Verification items for this drawing (mm, ordinates from the low corner). A direction names the side the tool comes from. Give positions to 0.01 mm unless a question says otherwise; leave off trailing zeros. Loops run counter-clockwise (first coordinate to the right, second up) from the corner with the lowest first, then second, coordinate; pieces in that order, holes last. Notation, with made-up numbers: (86.5, -5.75) -> (103.5, -5.75) arc R12 ccw to (103.5, 13.25) -> close; hole circle Ø4 at (-6.5, 81.5). An arc over 180 degrees is marked (long way). Write each question's results on one line, items separated by ' | '. Start each with the question number.
Item 1: Access from +Z, -Z, +X, -X, +Y, -Y to the whole of each face (thin tool, end or side, straight path). Record for the marked faces 1 and 2.
Item 2: Gauge pin test, flat end, axial feed: pin 1 Ø3 at (x, z) = (11, 19.5) entering from -Y. Record the tip position at first contact, or that the pin passes through.
Item 3: Mould release check, pull along Z, two halves, no side actions. Record for the marked faces 3, 4, 5 and 6: pulls with the +Z half, pulls with the -Z half, needs draft (parallel to the pull), parting line crosses it, or undercut.
Item 4: Cross-section at A-A on x = 12.5. Enter the section's corners in (y, z).
Item 5: Scan lines: line 1 along X through (y, z) = (6.35, 17.5); line 2 along X through (y, z) = (1.45, 17.5); line 3 along Z through (x, y) = (27.5, 2.5). Record each from-to range of solid material in increasing order.
Item 6: Cross-section at C-C on y = 0.5. Enter the section's corners in (x, z).
Item 7: Cross-section at B-B on z = 16.5. Enter the section's corners in (x, y).
Item 8: Cross-section at D-D on y = 7.75. Enter the section's corners in (x, z), then the cut area to 3 significant figures.
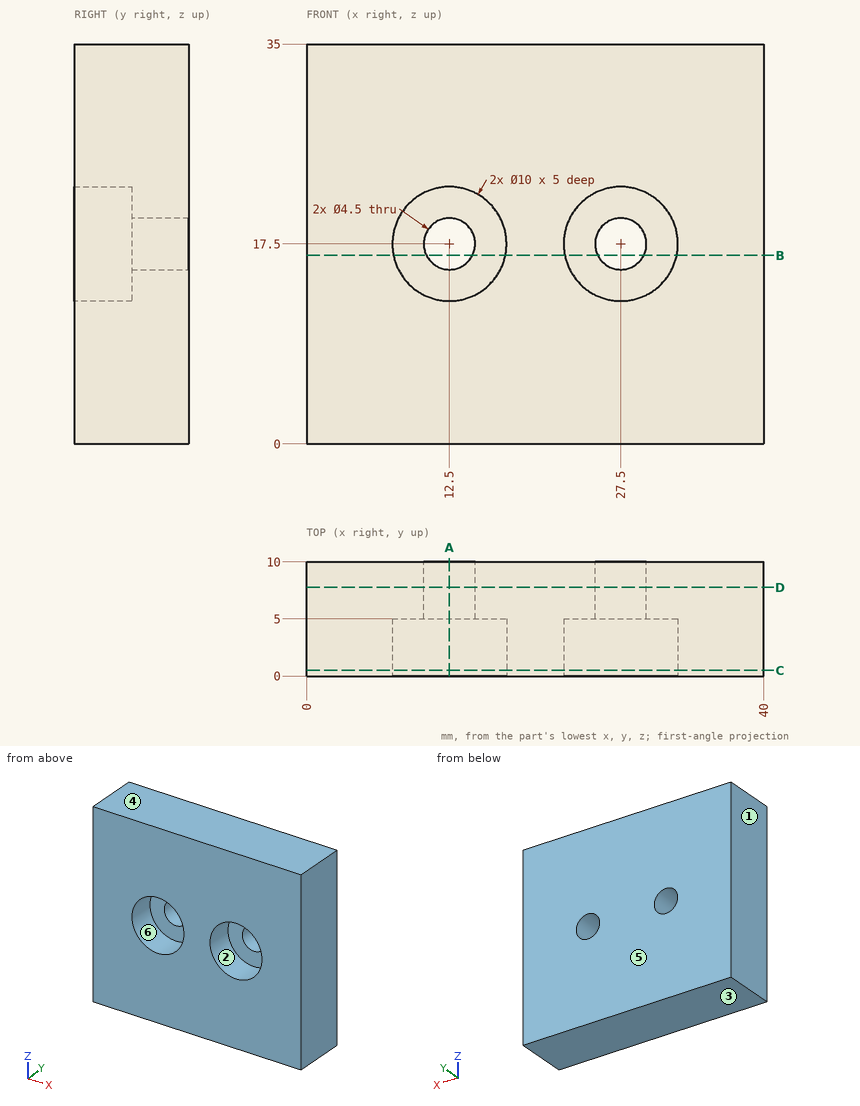
Answer sheet:
1) face 1: +Z, -Z, -X, +Y, -Y | face 2: -Y
2) pin 1: stops at y = 5
3) face 3: pulls with the -Z half | face 4: pulls with the +Z half | face 5: needs draft | face 6: undercut
4) outline: (0, 0) -> (10, 0) -> (10, 15.25) -> (5, 15.25) -> (5, 12.5) -> (0, 12.5) -> close; (0, 22.5) -> (5, 22.5) -> (5, 19.75) -> (10, 19.75) -> (10, 35) -> (0, 35) -> close
5) line 1: x = 0 to 10.25, 14.75 to 25.25, 29.75 to 40 | line 2: x = 0 to 7.5, 17.5 to 22.5, 32.5 to 40 | line 3: z = 0 to 12.5, 22.5 to 35
6) outline: (0, 0) -> (40, 0) -> (40, 35) -> (0, 35) -> close; hole circle Ø10 at (12.5, 17.5); hole circle Ø10 at (27.5, 17.5)
7) outline: (0, 0) -> (7.6, 0) -> (7.6, 5) -> (10.48, 5) -> (10.48, 10) -> (0, 10) -> close; (14.52, 5) -> (17.4, 5) -> (17.4, 0) -> (22.6, 0) -> (22.6, 5) -> (25.48, 5) -> (25.48, 10) -> (14.52, 10) -> close; (29.52, 5) -> (32.4, 5) -> (32.4, 0) -> (40, 0) -> (40, 10) -> (29.52, 10) -> close
8) outline: (0, 0) -> (40, 0) -> (40, 35) -> (0, 35) -> close; hole circle Ø4.5 at (12.5, 17.5); hole circle Ø4.5 at (27.5, 17.5) | area: 1,370 mm²
